Autodesk Inventor part; units mm, degrees
ref_plane "YZ Plane" through (0, 0, 0) normal (1, 0, 0) x (0, 1, 0)
ref_plane "XZ Plane" through (0, 0, 0) normal (0, 1, 0) x (-1, 0, 0)
ref_plane "XY Plane" through (0, 0, 0) normal (0, 0, 1) x (1, 0, 0)
sketch "Sketch1" plane through (0, 0, 0) normal (0, 0, 1) x (1, 0, 0)
  line L0 (5.9771, 0) -> (28.2021, 0)
  line L1 (28.2021, 0) -> (28.2021, 3.175)
  line L2 (28.2021, 3.175) -> (5.9771, 3.175)
  line L3 (2.8021, 6.35) -> (2.8021, 25.4)
  line L4 (5.9771, 28.575) -> (28.2021, 28.575)
  line L5 (28.2021, 28.575) -> (28.2021, 31.75)
  line L6 (28.2021, 31.75) -> (5.9771, 31.75)
  line L7 (-0.3729, 25.4) -> (-0.3729, 6.35)
  arc A0 (5.9771, 28.575) -> (2.8021, 25.4) centre (5.9771, 25.4) ccw
  arc A1 (2.8021, 6.35) -> (5.9771, 3.175) centre (5.9771, 6.35) ccw
  arc A2 (5.9771, 31.75) -> (-0.3729, 25.4) centre (5.9771, 25.4) ccw
  arc A3 (-0.3729, 6.35) -> (5.9771, 0) centre (5.9771, 6.35) ccw
  point P0 (0, 0)
  point P1 (-0.3729, 0)
  point P2 (2.8021, 3.175)
  point P3 (2.8021, 28.575)
  dimension "d0" = 28.575
  dimension "d1" = 3.175
  dimension "d2" = 25.4
  dimension "d3" = 25.4
  dimension "d4" = 3.175
  dimension "d5" = 3.175
  dimension "d6" = 6.35
extrude "Extrusion1" add sketch "Sketch1" against normal blind 889
sketch "Sketch2" plane through (-0.3729, 6.35, 0) normal (-1, 0, 0) x (0, 0, 1)
  line L0 (0, 19.05) -> (-889, 19.05)
  line L1 (-228.6, 0) -> (-228.6, 7.9375)
  arc A0 (-228.6, 11.1125) -> (-228.6, 7.9375) centre (-228.6, 9.525) ccw
  line L2 (-228.6, 11.1125) -> (-228.6, 19.05)
  line L3 (-228.6, 19.05) -> (-889, 19.05)
  line L4 (-889, 0) -> (-889, 19.05)
  line L5 (-889, 0) -> (-228.6, 0)
  circle A1 centre (-552.45, 11.43) radius 4.826
  circle A2 centre (-501.65, 11.43) radius 4.826
  circle A3 centre (-387.35, 11.43) radius 4.826
  circle A4 centre (-336.55, 11.43) radius 4.826
  circle A5 centre (-444.5, 7.62) radius 4.826
  circle A6 centre (-730.25, 11.43) radius 4.826
  circle A7 centre (-781.05, 11.43) radius 4.826
  line L6 (0, 25.4) -> (-889, 25.4) construction
  circle A8 centre (-133.35, 11.43) radius 4.826
  circle A9 centre (-82.55, 11.43) radius 4.826
  point P0 (0, -6.35)
  point P1 (-254, 0.852)
  dimension "d10" = 7.62
  dimension "d11" = 3.81
  dimension "d14" = 254
hole "Hole1" at (-0.3729, 17.78, -781.05) at (-0.3729, 17.78, -730.25) at (-0.3729, 17.78, -552.45) at (-0.3729, 17.78, -501.65) at (-0.3729, 13.97, -444.5) at (-0.3729, 17.78, -387.35) at (-0.3729, 17.78, -336.55) at (-0.3729, 17.78, -133.35) at (-0.3729, 17.78, -82.55) direction (1, 0, 0) diameter 9.652 end through all
hole "Hole2" at (-0.3729, 15.875, -228.6) direction (1, 0, 0) diameter 3.175 end through all
sketch "Sketch3" plane through (5.9771, 31.75, 0) normal (0, 1, 0) x (1, 0, 0)
  line L0 (22.225, 889) -> (0, 889)
  line L1 (22.225, 0) -> (22.225, 889)
  point P0 (-5.9771, 0)
  point P1 (9.525, 876.3)
  dimension "d34" = 12.7
  dimension "d35" = 12.7
hole "Hole3" at (15.5021, 31.75, -876.3) direction (0, -1, 0) diameter 6.5278 end through all
pattern_linear "Rectangular Pattern1" count 35 spacing 25.4 along (0, 0, 1) of "Hole3"
sketch "Sketch4" plane through (5.9771, 31.75, 0) normal (0, 1, 0) x (1, 0, 0)
  circle A0 centre (9.525, 12.7) radius 3.2639
  circle A1 centre (9.525, 38.1) radius 3.2639
  circle A2 centre (9.525, 63.5) radius 3.2639
  circle A3 centre (9.525, 88.9) radius 3.2639
  circle A4 centre (9.525, 114.3) radius 3.2639
  circle A5 centre (9.525, 139.7) radius 3.2639
  circle A6 centre (9.525, 165.1) radius 3.2639
  circle A7 centre (9.525, 190.5) radius 3.2639
  line L0 (22.225, 0) -> (-13.6032, 0)
  line L1 (-13.6032, 0) -> (-13.6032, 203.2)
  line L2 (-13.6032, 203.2) -> (22.225, 203.2)
  line L3 (22.225, 203.2) -> (22.225, 0)
  point P0 (-5.9771, 0)
  dimension "d46" = 203.2
extrude "Extrusion2" cut sketch "Sketch4" against normal blind 38.1
properties part number "chassis 27 inch"
Build history of the part. All positions in model axes, mm. A direction names the side the tool comes from. Round coordinates to 2 decimals unless told otherwise and drop trailing zeros. Write each loop counter-clockwise with the first axis right and the second up, starting at its lowest first coordinate (ties: lowest second). Pieces come first, ordered by that corner, then holes.
1) Pin check, flat tips, straight feed: pin 1 (1 mm diameter, centred on y = 4.5, z = -272.5, fed in from +X); pin 2 (6 mm diameter, centred on y = 16, z = -294, fed in from +X); pin 3 (4 mm diameter, centred on x = 15.5, z = -800.1, fed in from +Y). Stop position of each tip, or through.
2) Drill centre lines: probe 1 along Y at (x, z) = (14.25, -377) (3 decimals); probe 2 along X at (y, z) = (12, -857); probe 3 along Y at (x, z) = (3.5, -588). Where is each one in solid material? Low to high.
3) Band-saw the part on A-A, the plane z = -659. List the corners of the cut face in (x, y) (3 decimals).
4) Mould opens along Y. For faces 1 (the flat face through (17, 31.75, -541)), 2 (the flat face through (2, 15, -889)), 3 (the flat face through (17, 28.575, -541)) say: +Y half, -Y half, draft (parallel to the pull), parting line (faces both ways), or undercut.
5) 3-axis set-ups, long thin cutter, end or side, ignore diameter. For faces 4 (the flat face through (2.802, 16, -541)), 5 (the flat face through (2, 15, -203.2)): which of +Z, -Z, +X, -X, +Y, -Y reach the whole face in a straight line?
Ans:
1. pin 1: stops at x = 3.84
1. pin 2: stops at x = 2.8
1. pin 3: passes through
2. probe 1: y = 0 to 3.175, 28.575 to 31.75
2. probe 2: x = -0.37 to 2.8
2. probe 3: y = 0.5 to 4.36, 27.39 to 31.25
3. outline: (-0.373, 6.35) arc R6.35 ccw to (5.977, 0) - (28.202, 0) - (28.202, 3.175) - (5.977, 3.175) arc R3.175 cw to (2.802, 6.35) - (2.802, 25.4) arc R3.175 cw to (5.977, 28.575) - (28.202, 28.575) - (28.202, 31.75) - (5.977, 31.75) arc R6.35 ccw to (-0.373, 25.4) - close
4. face 1: +Y half
4. face 2: draft
4. face 3: undercut
5. face 4: +Z, -Z, +X
5. face 5: +Z, +X, -X, +Y, -Y
